Verification items for the finished model (mm, model axes). A direction names the side the tool comes from. Coordinates: 2 decimals unless noted, no trailing zeros. Write each loop counter-clockwise with the first axis right and the second up, starting at its lowest first coordinate (ties: lowest second). Pieces come first, ordered by that corner, then holes. Notation, with made-up numbers: (-20.75, 70) - (18.25, 70) arc R11 ccw to (18.25, 89) - close; hole circle Ø5 at (32, -4). An arc over 180 degrees is marked (long way). Use CSV: the item, a comma, the result in double quotes. Start each with the question number.
```python
from build123d import *

# Parameters (mm, degrees)
BOSS_EXTRUDE1_DEPTH = 12
SKETCH2_R           = 2.1
CUT_EXTRUDE1_DEPTH  = 8


with BuildPart() as part:
    # Sketch1 → Boss-Extrude1 (new body)
    with BuildSketch(Plane.XY):
        with BuildLine():
            Line((1.021227299, 0), (4.978772701, 0))
            ThreePointArc((4.978772701, 0), (5.700889449, 0.299110551), (6, 1.021227299))
            Line((6, 1.021227299), (6, 5.978772701))
            ThreePointArc((6, 5.978772701), (5.700889449, 6.700889449), (4.978772701, 7))
            Line((4.978772701, 7), (1.021227299, 7))
            ThreePointArc((1.021227299, 7), (0.299110551, 6.700889449), (0, 5.978772701))
            Line((0, 5.978772701), (0, 1.021227299))
            ThreePointArc((0, 1.021227299), (0.299110551, 0.299110551), (1.021227299, 0))
        make_face()
    extrude(amount=BOSS_EXTRUDE1_DEPTH)

    # Sketch2 → Cut-Extrude1 (cut)
    with BuildSketch(Plane.XY.offset(12)):
        with Locations((3, 3.5)):
            Circle(SKETCH2_R)
    extrude(amount=-CUT_EXTRUDE1_DEPTH, mode=Mode.SUBTRACT)


solid = part.part
```
Q1. Tool access check on faces 4 (the flat face through (3, 7, 6)), 5 (the cylindrical face through (3.969, 1.637, 8.056)). Record the directions out of +Z, -Z, +X, -X, +Y, -Y that give a thin tool (end or side, any length) a straight path to the whole face; none if there is none.
Q2. Release check for a two-part mould opening along X. For faces 1 (the flat face through (3, 6, 12)), 2 (the flat face through (3, 4, 4)), 3 (the cylindrical face through (5.7, 0.3, 5.9)) record: released by +X, released by -X, zero draft, split by the parting line, or undercut.
Q3. Cross-section at B-B (z = 4.75). Record the cut outline in (x, y).
Q4. Cross-section at C-C (y = 3.5). Record the cut outline in (x, z), plus the area to 3 significant figures.
Q5. Gauge pin test, flat end, axial feed: pin 1 (3.5 mm diameter, centred on x = 3, y = 3.5, fed in from +Z). Record the tip position at first contact, or that the pin passes through.
Q6. Cross-section at A-A (x = 3). Record the cut outline in (y, z).
Q7. Scan lines: line 1 along Y through (x, z) = (3, 8); line 2 along Z through (x, y) = (4.35, 3.5); line 3 along Y through (x, z) = (3.65, 9.75). Record each from-to range of solid material in increasing order. Write a range as from..to.
Reply:
1,face 4,"+Z, -Z, +X, -X, +Y"
1,face 5,"+Z"
2,face 1,"zero draft"
2,face 2,"undercut"
2,face 3,"released by +X"
3,outline,"(0, 1.02) arc R1.02 ccw to (1.02, 0) - (4.98, 0) arc R1.02 ccw to (6, 1.02) - (6, 5.98) arc R1.02 ccw to (4.98, 7) - (1.02, 7) arc R1.02 ccw to (0, 5.98) - close; hole circle Ø4.2 at (3, 3.5)"
4,outline,"(0, 0) - (6, 0) - (6, 12) - (5.1, 12) - (5.1, 4) - (0.9, 4) - (0.9, 12) - (0, 12) - close"
4,area,"38.4 mm^2"
5,pin 1,"z = 4"
6,outline,"(0, 0) - (7, 0) - (7, 12) - (5.6, 12) - (5.6, 4) - (1.4, 4) - (1.4, 12) - (0, 12) - close"
7,line 1,"0..1.4, 5.6..7"
7,line 2,"0..4"
7,line 3,"0..1.5, 5.5..7"
